Part model, mm, in its own coordinate system. Face numbers are marked on the shaded views. A direction names the side the tool comes from. Give positions to 0.01 mm unless a question says otherwise; leave off trailing zeros. Write each loop counter-clockwise with the first axis right and the second up, starting at its lowest first coordinate (ties: lowest second). Pieces come first, ordered by that corner, then holes.
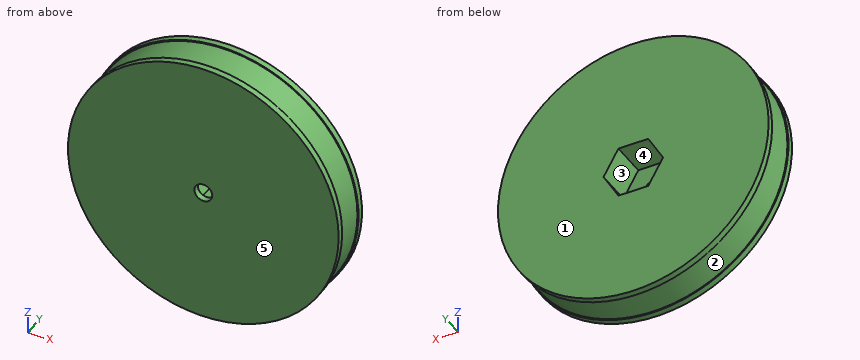
Autodesk Fusion 360 part; units mm, degrees
sketch "spodek" plane through (0, 0, 0) normal (0, 1, 0) x (1, 0, 0)
  circle A0 centre (0, 0) radius 31.75
  circle A1 centre (0, 0) radius 2.1
  dimension "d1" = 63.5
  dimension "d2" = 4.2
extrude "Extrude1" add sketch "spodek" along normal blind 1.5
sketch "prostredek" plane through (0, 1.5, 0) normal (0, 1, 0) x (-1, 0, 0)
  circle A0 centre (0, 0) radius 2.1
  circle A1 centre (0, 0) radius 31.75
  circle A2 centre (0, 0) radius 31.5
  line L0 (3.493, -6.05) -> (6.9859, 0)
  line L1 (6.9859, 0) -> (3.493, 6.05)
  line L2 (3.493, 6.05) -> (-3.493, 6.05)
  line L3 (-3.493, 6.05) -> (-6.9859, 0)
  line L4 (-6.9859, 0) -> (-3.493, -6.05)
  line L5 (-3.493, -6.05) -> (3.493, -6.05)
  dimension "d5" = -0.25
  dimension "d6" = 6.05
extrude "Extrude2" add sketch "prostredek" along normal blind 7 contours A2
sketch "Sketch3" plane through (0, 8.5, 0) normal (0, 1, 0) x (-1, 0, 0)
  line L0 (3.493, -6.05) -> (-3.493, -6.05)
  line L1 (-3.493, -6.05) -> (-6.9859, 0)
  line L2 (-6.9859, 0) -> (-3.493, 6.05)
  line L3 (-3.493, 6.05) -> (3.493, 6.05)
  line L4 (3.493, 6.05) -> (6.9859, 0)
  line L5 (6.9859, 0) -> (3.493, -6.05)
  line L6 (-6.9859, 0) -> (-3.493, 6.05)
  line L7 (-3.493, -6.05) -> (-6.9859, 0)
  line L8 (3.493, -6.05) -> (-3.493, -6.05)
  line L9 (6.9859, 0) -> (3.493, -6.05)
  line L10 (-3.493, 6.05) -> (3.493, 6.05)
  circle A0 centre (0, 0) radius 31.75
extrude "Extrude3" add sketch "Sketch3" along normal blind 1.5
1) 3-axis set-ups, long thin cutter, end or side, ignore diameter. For the marked faces 4 and 5: which of +Z, -Z, +X, -X, +Y, -Y reach the whole face in a straight line?
Answers follow:
face 4: +Y
face 5: +Z, -Z, +X, -X, -Y
2) Saw through at C-C, the plane x = 11. Write the cut outline in (y, z).
Answers follow:
outline: (0, -29.78) - (1.5, -29.78) - (1.5, -29.52) - (8.5, -29.52) - (8.5, -29.78) - (10, -29.78) - (10, 29.78) - (8.5, 29.78) - (8.5, 29.52) - (1.5, 29.52) - (1.5, 29.78) - (0, 29.78) - close
3) Pin check, flat tips, straight feed: pin 1 Ø3 at (y, z) = (6, 15) entering from -X; pin 2 Ø1 at (x, y) = (4, 5) entering from -Z; pin 3 Ø1 at (y, z) = (3, 18) entering from +X. Stop position of each tip, or through.
Answers follow:
pin 1: stops at x = -28.46
pin 2: stops at z = -31.3
pin 3: stops at x = 26.19
4) Two-plate mould, pull along Z, no slides. Class the marked faces 1, 2 and 3: +Z half, -Z half, draft (parallel to the pull), parting line (faces both ways), or undercut.
Answers follow:
face 1: draft
face 2: parting line
face 3: undercut
5) Wall check: L1, parallel to X at y = 0.3, z = 0; L2, parallel to X at y = 1, z = 1. Give the ranges that are in metal, low to high.
Answers follow:
L1: x = -31.75 to -2.1, 2.1 to 31.75
L2: x = -31.73 to -1.85, 1.85 to 31.73
6) Saw through at B-B, the plane z = -10.5. Write the cut outline in (x, y), then the cut area to 3 significant figures.
Answers follow:
outline: (-29.96, 0) - (29.96, 0) - (29.96, 1.5) - (29.7, 1.5) - (29.7, 8.5) - (29.96, 8.5) - (29.96, 10) - (-29.96, 10) - (-29.96, 8.5) - (-29.7, 8.5) - (-29.7, 1.5) - (-29.96, 1.5) - close
area: 596 mm2
7) Saw through at A-A, the plane x = 0. Write the cut outline in (y, z), then the cut area to 3 significant figures.
Answers follow:
outline: (0, -31.75) - (1.5, -31.75) - (1.5, -31.5) - (8.5, -31.5) - (8.5, -31.75) - (10, -31.75) - (10, -6.05) - (1.5, -6.05) - (1.5, -2.1) - (0, -2.1) - close; (0, 2.1) - (1.5, 2.1) - (1.5, 6.05) - (10, 6.05) - (10, 31.75) - (8.5, 31.75) - (8.5, 31.5) - (1.5, 31.5) - (1.5, 31.75) - (0, 31.75) - close
area: 522 mm2
